Source: three-view drawing plus pictorial views. Frame: mm from the lowest corner of the part. Give positions to 0.01 mm unless a question says otherwise; leave off trailing zeros. Order: outer loops, then holes, each group sorted by start corner. A loop starts at its lowest first (then second) coordinate and runs counter-clockwise, first axis right, second up. Notation, with made-up numbers: (21, 70.5) - (57, 70.5) arc R7 ccw to (57, 76.5) - close; hole circle Ø7 at (14.5, 9). An arc over 180 degrees is marked (long way). Use one line per item in the form item = value.
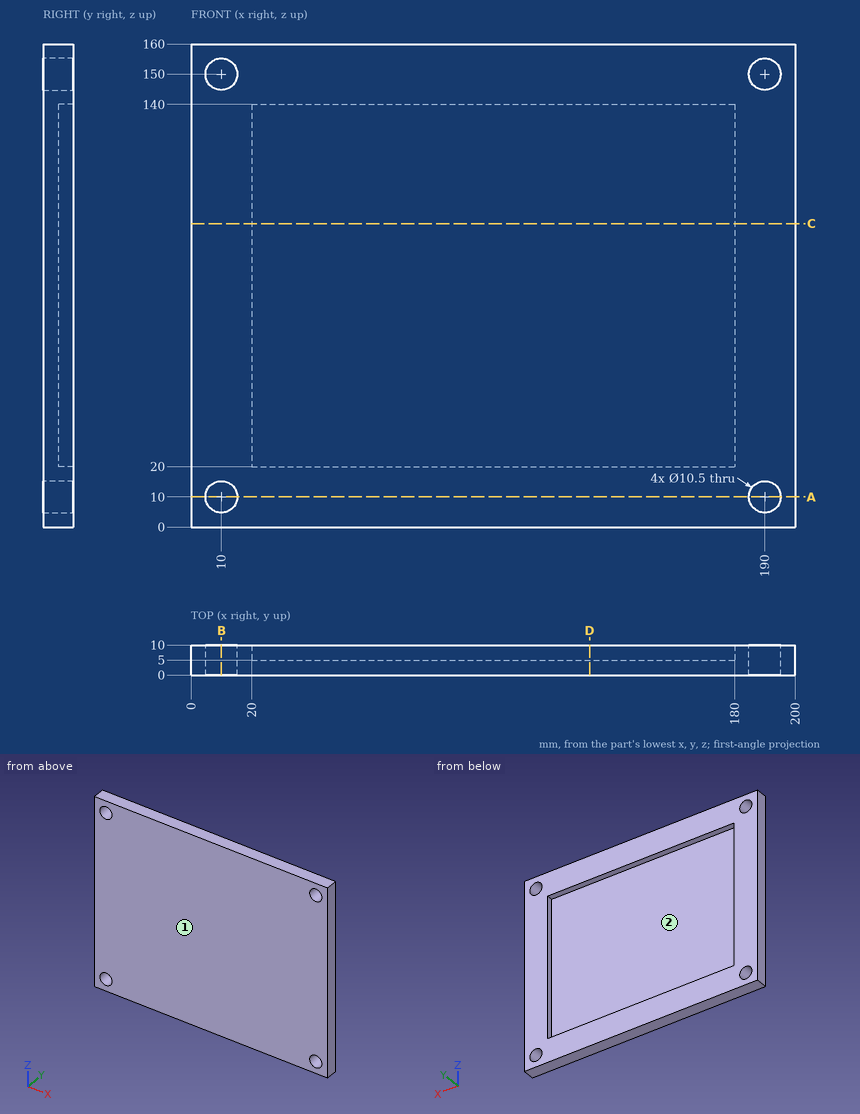
(1) Cut plane C-C on z = 100.5. Output: boundary loops of the cut face in (x, y), plus the area to 3 significant figures.
Computed values:
outline = (0, 0) - (200, 0) - (200, 10) - (180, 10) - (180, 5) - (20, 5) - (20, 10) - (0, 10) - close
area = 1,200 mm²
(2) Cut plane D-D on x = 132. Output: boundary loops of the cut face in (y, z), plus the area to 3 significant figures.
Computed values:
outline = (0, 0) - (10, 0) - (10, 20) - (5, 20) - (5, 140) - (10, 140) - (10, 160) - (0, 160) - close
area = 1,000 mm²
(3) Cut plane B-B on x = 10. Output: boundary loops of the cut face in (y, z).
Computed values:
outline = (0, 0) - (10, 0) - (10, 4.75) - (0, 4.75) - close; (0, 15.25) - (10, 15.25) - (10, 144.75) - (0, 144.75) - close; (0, 155.25) - (10, 155.25) - (10, 160) - (0, 160) - close
(4) Cut plane A-A on z = 10. Output: boundary loops of the cut face in (x, y), plus the area to 3 significant figures.
Computed values:
outline = (0, 0) - (4.75, 0) - (4.75, 10) - (0, 10) - close; (15.25, 0) - (184.75, 0) - (184.75, 10) - (15.25, 10) - close; (195.25, 0) - (200, 0) - (200, 10) - (195.25, 10) - close
area = 1,790 mm²
(5) Ray query, line 1 along X through (y, z) = (5, 150); line 2 along X through (y, z) = (5.5, 58); line 3 along Z through (x, y) = (14.5, 6). Return the intervals inside material, ascending.
Computed values:
line_1 = 0 to 4.75, 15.25 to 184.75, 195.25 to 200
line_2 = 0 to 20, 180 to 200
line_3 = 0 to 7.3, 12.7 to 147.3, 152.7 to 160
(6) Pull-direction query (Z, two-part tool) for the marked faces 1 and 2; classes: released by +Z, released by -Z, zero draft, split by the parting line, or undercut.
Computed values:
face_1 = zero draft
face_2 = undercut
(7) Contact query for flat-ended pins moving along their axis: pin 1 Ø6.5 at (x, z) = (190, 10) entering from -Y; pin 2 Ø3 at (x, z) = (46, 81) entering from +Y. Output: stop coordinate, or through.
Computed values:
pin_1 = through
pin_2 = 5
